Work out the finished part from the listing and answer in its coordinate system (mm). Round coordinates to 2 decimals unless told otherwise and drop trailing zeros. Write each loop counter-clockwise with the first axis right and the second up, starting at its lowest first coordinate (ties: lowest second). Pieces come first, ordered by that corner, then holes.
1. Find section A-A (z = 25). Count the separate pieces of the cut face and the enclosed holes in it, and give its area (3 significant figures).
2. Flat-ended cylindrical pins translate along their axes: pin 1 Ø3 at (x, y) = (-178.5, 1.5) entering from -Z; pin 2 Ø3 at (x, y) = (-106.5, -1) entering from -Z. Find the tip coordinate at first contact, or state that the pin passes through.
3. Find section B-B (y = -1). Write down the section's boundary in (x, z).
4. Find section C-C (x = -90). Write down the section's boundary in (y, z), and give its area (3 significant figures).
5. Straight lines are drawn through the part: probe 1 along X at (y, z) = (0.75, 45); probe 2 along Z at (x, y) = (-268, 0.75); probe 3 along Z at (x, y) = (-237, 2). For each, find the intervals that lie inside material, in ascending order.
Autodesk Inventor part; units mm, degrees
ref_plane "YZ Plane" through (0, 0, 0) normal (1, 0, 0) x (0, 1, 0)
ref_plane "XZ Plane" through (0, 0, 0) normal (0, 1, 0) x (-1, 0, 0)
ref_plane "XY Plane" through (0, 0, 0) normal (0, 0, 1) x (1, 0, 0)
sketch "Sketch1" plane through (0, 0, 0) normal (0, 0, 1) x (1, 0, 0)
  circle A0 centre (0, 0) radius 400 construction
  line L0 (-399, 5) -> (399, 5)
  line L1 (399, 5) -> (399, -5)
  line L2 (399, -5) -> (-399, -5)
  line L3 (-399, -5) -> (-399, 5)
  line L4 (-399, 5) -> (399, -5) construction
  dimension "d0" = 800
  dimension "d1" = 10
  dimension "d2" = 798
extrude "Extrusion1" add sketch "Sketch1" along normal blind 100
sketch "Sketch2" plane through (-399, -5, 0) normal (0, -1, 0) x (1, 0, 0)
  circle A0 centre (309, 0) radius 40
  line L0 (0, 0) -> (798, 0)
  circle A1 centre (129, 0) radius 40
  circle A2 centre (489, 0) radius 40
  circle A3 centre (669, 0) radius 40
  line L1 (394, 50) -> (404, 50)
  line L2 (404, 50) -> (404, 0)
  line L3 (404, 0) -> (394, 0)
  line L4 (394, 0) -> (394, 50)
  line L5 (214, 50) -> (224, 50)
  line L6 (224, 50) -> (224, 0)
  line L7 (224, 0) -> (214, 0)
  line L8 (214, 0) -> (214, 50)
  line L9 (574, 50) -> (584, 50)
  line L10 (584, 50) -> (584, 0)
  line L11 (584, 0) -> (574, 0)
  line L12 (574, 0) -> (574, 50)
  point P0 (399, 0)
  point P1 (399, 0)
  point P2 (399, 0)
  point P3 (399, 0)
  point P4 (709, 0)
  point P5 (629, 0)
  point P6 (529, 0)
  point P7 (449, 0)
  point P8 (269, 0)
  point P9 (349, 0)
  point P10 (169, 0)
  point P11 (89, 0)
  point P12 (399, 0)
  point P13 (219, 0)
  point P14 (399, 0)
  point P15 (399, 0)
  point P16 (579, 0)
  point P17 (399, 0)
  point P18 (399, 0)
  point P19 (574, 0)
  point P20 (584, 0)
  point P21 (214, 0)
  point P22 (224, 0)
  dimension "d5" = 80
  dimension "d7" = 90
  dimension "d8" = 80
  dimension "d9" = 180
  dimension "d10" = 80
  dimension "d11" = 80
  dimension "d12" = 90
  dimension "d13" = 180
  dimension "d24" = 10
  dimension "d25" = 50
  dimension "d26" = 10
  dimension "d27" = 50
  dimension "d28" = 180
  dimension "d29" = 10
  dimension "d30" = 50
  dimension "d31" = 180
extrude "Extrusion2" cut sketch "Sketch2" against normal through all contours L0 A0 | L0 A1 | L0 L8 L5 L6 | A3 L0 | L12 L9 L10 L0 | A2 L0 | L4 L1 L2 L0 picked at (302.3333, 20.5179) picked at (130.5738, 20.5179) picked at (658.2131, 7.8371) picked at (497.9217, 9.9086)
equation "\"d26\" = d24"
equation "\"d27\" = d25"
equation "\"d29\" = d24"
equation "\"d30\" = d25"
equation "\"BendReliefWidth\" = Thickness"
equation "\"BendReliefDepth\" = 0.5 * Thickness"
equation "\"CornerReliefSize\" = 4 * Thickness"
equation "\"MinimumRemnant\" = 2 * Thickness"
equation "\"TransitionRadius\" = BendRadius"
equation "\"JacobiRadiusSize\" = BendRadius"
equation "\"GapSize\" = Thickness"
properties part number "BSH 084 amplifier bottom" material "Stainless Steel"
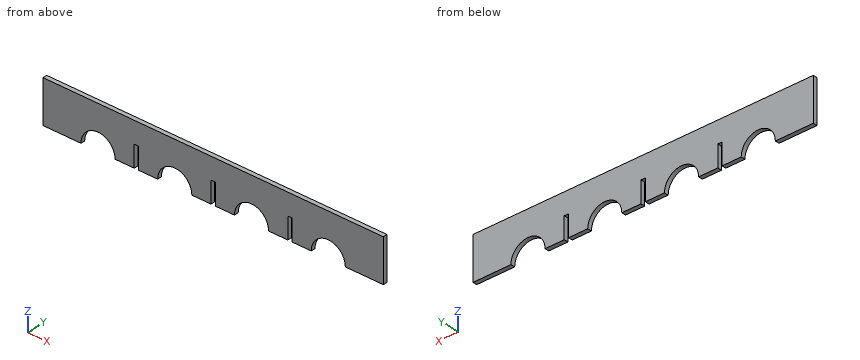
Worked answers:
1. separate pieces: 8
1. enclosed holes: 0
1. area: 5,180 mm2
2. pin 1: stops at z = 50
2. pin 2: stops at z = 35.72
3. outline: (-399, 0) - (-310, 0) arc R40 cw to (-230, 0) - (-185, 0) - (-185, 50) - (-175, 50) - (-175, 0) - (-130, 0) arc R40 cw to (-50, 0) - (-5, 0) - (-5, 50) - (5, 50) - (5, 0) - (50, 0) arc R40 cw to (130, 0) - (175, 0) - (175, 50) - (185, 50) - (185, 0) - (230, 0) arc R40 cw to (310, 0) - (399, 0) - (399, 100) - (-399, 100) - close
4. outline: (-5, 40) - (5, 40) - (5, 100) - (-5, 100) - close
4. area: 600 mm2
5. probe 1: x = -399 to -185, -175 to -5, 5 to 175, 185 to 399
5. probe 2: z = 39.95 to 100
5. probe 3: z = 22.61 to 100
